For this review, take the finished solid that the model builds, in its own axes (mm). Give positions to 0.01 mm unless a question says otherwise; leave off trailing zeros. Write each loop counter-clockwise with the first axis right and the second up, starting at its lowest first coordinate (ties: lowest second). Pieces come first, ordered by that corner, then holes. Notation, with made-up numbers: (-33.75, 66) -> (14.25, 66) arc R32 cw to (14.25, 99) -> close; hole circle Ø1 at (5, 55). An arc over 180 degrees is marked (long way). Return JSON: item names as keys, results as strings.
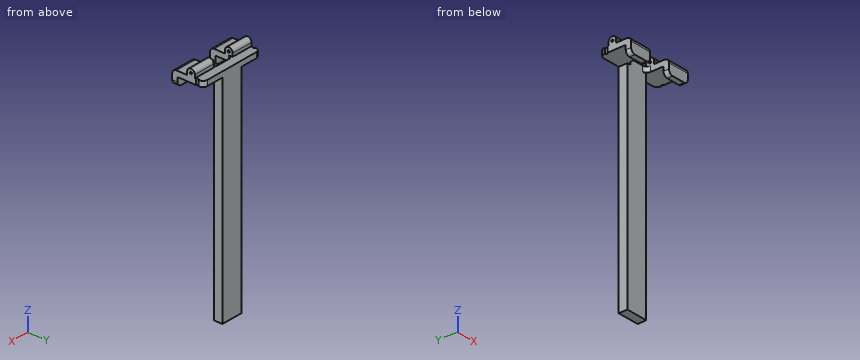
from build123d import *

# Parameters (mm, degrees)
F0_W     = 5
F0_H     = 4
F1_DEPTH = 101.6
F2_R     = 0.5
F3_DEPTH = 10
F4_R     = 2
F5_R     = 0.5
F7_DEPTH = 101.601


with BuildPart() as f1:
    # F0 (on Top) → F1 (new body)
    with BuildSketch(Plane.XY):
        with Locations((2.5, -2)):
            Rectangle(F0_W, F0_H)
    extrude(amount=-F1_DEPTH)

    # F2 (on face) → F3 (join)
    with BuildSketch(Plane.YZ.offset(5)):
        with BuildLine():
            Line((0, -2.5), (0, 0))
            Line((0, 0), (-4, 0))
            Line((-4, 0), (-4, 1.5))
            ThreePointArc((-4, 1.5), (-5.7784285378, 3.2784285378), (-7.5568570755, 1.5))
            Line((-7.5568570755, 1.5), (-7.5568570755, 0))
            Line((-7.5568570755, 0), (-14.5, 0))
            Line((-14.5, 0), (-14.5, -6.5))
            Line((-14.5, -6.5), (-12, -6.5))
            Line((-12, -6.5), (-12, -2.5))
            Line((-12, -2.5), (0, -2.5))
        make_face()
        with Locations((-5.7784285378, 1.5)):
            Circle(F2_R, mode=Mode.SUBTRACT)
    extrude(amount=F3_DEPTH)

    # F4
    f4_edges = [f1.edges().sort_by_distance(p)[0] for p in [
        (10, -14.5, 0),
        (5, -4, -1.25),
        (15, 0, -1.25),
        (15, -13.25, -6.5),
        (5, -13.25, -6.5),
    ]]
    fillet(f4_edges, radius=F4_R)

    # F5
    f5_edges = [f1.edges().sort_by_distance(p)[0] for p in [
        (10, -12, -2.5),
    ]]
    fillet(f5_edges, radius=F5_R)

    # F6 (on face) → F7 (cut, through all)
    with BuildSketch(Plane.XY):
        with BuildLine():
            Line((15, -3.4615779296), (15, -2.3238305002))
            ThreePointArc((15, -2.3238305002), (14.4311262853, -2.8927042149), (15, -3.4615779296))
        make_face()
    extrude(amount=-F7_DEPTH, mode=Mode.SUBTRACT)

    # F8: F1 across plane


with BuildPart() as f1_1:
    add(f1.part)
    add(f1.part.mirror(Plane.YZ))


solid = f1_1.part
1. Add section A-A, the plane x = -10.25. State the section outline as (y, z) points, plus the area to 3 significant figures.
Results found:
{"outline": "(-14.5, -6.5) -> (-12, -6.5) -> (-12, -3) arc R0.5 cw to (-11.5, -2.5) -> (0, -2.5) -> (0, 0) -> (-4, 0) -> (-4, 1.5) arc R1.78 ccw to (-7.56, 1.5) -> (-7.56, 0) -> (-12.5, 0) arc R2 ccw to (-14.5, -2) -> close; hole circle Ø1 at (-5.78, 1.5)", "area": "55.0 mm²"}
2. Add section C-C, the plane x = 1.75. State the section outline as (y, z) points, plus the area to 3 significant figures.
Results found:
{"outline": "(-4, -101.6) -> (0, -101.6) -> (0, 0) -> (-4, 0) -> close", "area": "406 mm²"}
3. Add section B-B, the plane z = -44. State the section outline as (x, y) points.
Results found:
{"outline": "(-5, -4) -> (5, -4) -> (5, 0) -> (-5, 0) -> close"}
4. For pin 1 (3 mm diameter, centred on x = 11.5, y = -3, fed in from -Z); pin 2 (8 mm diameter, centred on x = -7, y = -5.5, fed in from +Z); pin 3 (5 mm diameter, centred on y = -3.5, z = -30, fed in from -X); pin 4 (5 mm diameter, centred on x = 0, z = -70.5, fed in from -Y), all flat-tipped, find the tip position at first contact; note any pin that passes through.
Results found:
{"pin 1": "stops at z = -2.5", "pin 2": "stops at z = 3.28", "pin 3": "stops at x = -5", "pin 4": "stops at y = -4"}
5. To check wall thickness, follow probe 1 along Z at (x, y) = (-10.75, -3); probe 2 along Z at (x, y) = (-6.75, -5.75); probe 3 along Z at (x, y) = (11.5, -12.5). State the ranges of each line that lie inside material, in increasing order.
Results found:
{"probe 1": "z = -2.5 to 0", "probe 2": "z = -2.5 to 1, 2 to 3.28", "probe 3": "z = -6.5 to 0"}
